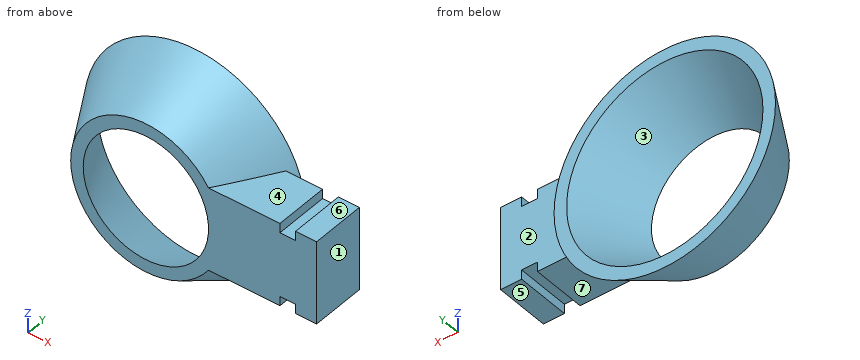
```python
from build123d import *

# Parameters (mm, degrees)
F3_W     = 8.786383085
F3_H     = 13.5255949572
F5_DEPTH = 10.16
F6_W     = 2.54
F6_H     = 8.786383085
F7_DEPTH = 1.524


# Not quite as in the source:
# - a pattern or mirror of a feature is missing from the dataset's text; its kind, count and spacing are read off the source's solid


with BuildPart() as f1:
    # F0 (on Top) → F1 (revolve)
    with BuildSketch(Plane.XY):
        Polygon((-12.192, 0), (-10.16, 0), (-15.9150013827, 10.16), (-17.9470013827, 10.16), align=None)
    revolve(axis=Axis((0, 4.3423168827, 0), (0, -1, 0)))

    # F3 (on offset) → F4 (join, up to the next surface of F1)
    with BuildSketch(Plane.YZ.offset(17.526)):
        with Locations((4.3931915425, 0)):
            Rectangle(F3_W, F3_H)
    extrude(until=Until.NEXT, dir=(-1, 0, 0))

    # F5 (add): a face of the model
    f5_faces = [f1.faces().sort_by_distance(p)[0] for p in [
        (17.526, 4.3931915425, 0),
    ]]
    extrude(f5_faces, amount=F5_DEPTH)

    # F6 (on face) → F7 (cut)
    with BuildSketch(Plane.XY.offset(6.7627974786)):
        with Locations((23.0034508117, 4.3931915425)):
            Rectangle(F6_W, F6_H)
    f7 = extrude(amount=-F7_DEPTH, mode=Mode.SUBTRACT)

    # F7_copies: F7 across plane
    add(f7.mirror(Plane(origin=(0, 0, 0), x_dir=(-1, 0, 0), z_dir=(0, 0, -1))), mode=Mode.SUBTRACT)


solid = f1.part
```
Geometry: final body of the model. Coordinates: model frame, mm. Face numbers are marked on the shaded views. A direction names the side the tool comes from. Coordinates: 2 decimals unless noted, no trailing zeros. Order: outer loops, then holes, each group sorted by start corner. A loop starts at its lowest first (then second) coordinate and runs counter-clockwise, first axis right, second up. Notation, with made-up numbers: M -38.5,3 L 14.5,3 A16 ccw 14.5,34 Z; hole C 87,51.5 d3. An arc over 180 degrees is marked long. Answer in a Markdown table with one row per item. Add a question column.
Q1. Reachability of the marked faces 4, 5, 6 and 7 from +Z, -Z, +X, -X, +Y, -Y: full face, straight path, thin tool, end or side. Return the list, or none.
Q2. Section query C-C on y = 5.5. Return the cut outline in (x, z), and give its area (3 significant figures).
Q3. Section query B-B on z = 0. Return the cut outline in (x, y) (3 decimals), and give its area (3 significant figures).
Q4. Mould query, pull axis X, two halves, no side actions, for the marked faces 1, 2 and 3. Classes: released by +X, released by -X, zero draft, split by the parting line, or undercut.
Q5. Contact query for flat-ended pins moving along their axis: P1, Ø6, axis at x = 8, z = -5.5, coming from the +Y side; P2, Ø6, axis at x = -12.5, y = 8, coming from the +Z side; P3, Ø5, axis at x = 8.5, z = 6.5, coming from the +Y side; P4, Ø6, axis at x = 18.5, z = -2, coming from the -Y side. Output: stop coordinate, or through.
Q6. Section query A-A on x = 0. Return the cut outline in (y, z) (3 decimals).
Q7. Section query D-D on y = 1.75. Return the cut outline in (x, z).
Q8. Line query: L1, parallel to X at y = 1.75, z = -6; L2, parallel to Z at x = 24, y = 7.5; L3, parallel to X at y = 5, z = 7.5. Output: solid intervals per line, ascending.
Completed:
| question | item | result |
|---|---|---|
| 1 | face 4 | +Z, +X, -Y |
| 1 | face 5 | -Z, +X, +Y, -Y |
| 1 | face 6 | +Z, +X, +Y, -Y |
| 1 | face 7 | -Z, +X, -Y |
| 2 | outline | M 13.73,-6.76 L 21.73,-6.76 L 21.73,-5.24 L 24.27,-5.24 L 24.27,-6.76 L 27.69,-6.76 L 27.69,6.76 L 24.27,6.76 L 24.27,5.24 L 21.73,5.24 L 21.73,6.76 L 13.73,6.76 A15.31 ccw long Z; hole C 0,0 d26.55 |
| 2 | area | 349 mm2 |
| 3 | outline | M -17.947,10.16 L -12.192,0 L -10.16,0 L -15.915,10.16 Z; M 10.16,0 L 27.686,0 L 27.686,8.786 L 17.169,8.786 L 17.947,10.16 L 15.915,10.16 Z |
| 3 | area | 156 mm2 |
| 4 | face 1 | released by +X |
| 4 | face 2 | zero draft |
| 4 | face 3 | undercut |
| 5 | P1 | stops at y = 4.5 |
| 5 | P2 | stops at z = 14.61 |
| 5 | P3 | stops at y = 5.37 |
| 5 | P4 | stops at y = 0 |
| 6 | outline | M 0,-12.192 L 10.16,-17.947 L 10.16,-15.915 L 0,-10.16 Z; M 0,10.16 L 10.16,15.915 L 10.16,17.947 L 0,12.192 Z |
| 7 | outline | M 11.32,-6.76 L 21.73,-6.76 L 21.73,-5.24 L 24.27,-5.24 L 24.27,-6.76 L 27.69,-6.76 L 27.69,6.76 L 24.27,6.76 L 24.27,5.24 L 21.73,5.24 L 21.73,6.76 L 11.32,6.76 A13.18 ccw long Z; hole C 0,0 d22.3 |
| 8 | L1 | x = -11.74 to -9.4, 9.4 to 21.73, 24.27 to 27.69 |
| 8 | L2 | z = -5.24 to 5.24 |
| 8 | L3 | x = -13.02 to -10.61, 10.61 to 13.02 |
